Autodesk Inventor part; units mm, degrees
ref_plane "YZ Plane" through (0, 0, 0) normal (1, 0, 0) x (0, 1, 0)
ref_plane "XZ Plane" through (0, 0, 0) normal (0, 1, 0) x (-1, 0, 0)
ref_plane "XY Plane" through (0, 0, 0) normal (0, 0, 1) x (1, 0, 0)
sketch "Sketch1" plane through (0, 0, 0) normal (0, 1, 0) x (-1, 0, 0)
  line L0 (0, 0) -> (152.4, 0)
  line L1 (152.4, 0) -> (152.4, -762)
  line L2 (0, -762) -> (0, 0)
  line L3 (152.4, -762) -> (0, -762) construction
  arc A0 (0, -762) -> (152.4, -762) centre (76.2, -936.5961) ccw
  line L4 (152.4, -590.1365) -> (152.4, -762) construction
  arc A1 (12.7, -770.5221) -> (139.7, -770.5221) centre (76.2, -936.5961) ccw
  line L5 (12.7, -12.7) -> (139.7, -12.7)
  line L6 (139.7, -12.7) -> (139.7, -749.3)
  line L7 (12.7, -749.3) -> (12.7, -12.7)
  line L8 (12.7, -12.7) -> (139.7, -749.3) construction
  line L9 (139.7, -12.7) -> (12.7, -749.3) construction
  line L10 (12.7, -749.3) -> (12.7, -770.5221)
  line L11 (139.7, -749.3) -> (139.7, -770.5221)
  point P0 (76.2, -381)
  dimension "d0" = 762
  dimension "d1" = 381
  dimension "d2" = 355.6
  dimension "d3" = 762
  dimension "d4" = 127
  dimension "d5" = 736.6
extrude "Extrusion1" add sketch "Sketch1" along normal blind 12.7
properties part number "Arm Layer 2 Out"
For this review, take the finished solid that the model builds, in its own axes (mm). Round coordinates to 2 decimals unless told otherwise and drop trailing zeros. Write each loop counter-clockwise with the first axis right and the second up, starting at its lowest first coordinate (ties: lowest second). Pieces come first, ordered by that corner, then holes. Notation, with made-up numbers: (54, 44.25) - (103, 44.25) arc R31 cw to (103, 73.25) - close; hole circle Ø10 at (40, 75). An arc over 180 degrees is marked (long way). Use CSV: the item, a comma, the result in double quotes.
1) Add section C-C on y = 4.75. Write out the cut boundary in (x, z), and give its area (3 significant figures).
Conclusion:
outline,"(-152.4, -762) arc R190.5 ccw (long way) to (0, -762) - (0, 0) - (-152.4, 0) - close; hole (-139.7, -770.52) arc R177.8 ccw (long way) to (-12.7, -770.52) - (-12.7, -12.7) - (-139.7, -12.7) - close"
area,"33,900 mm^2"
2) Add section B-B on x = -76.2. Write out the cut boundary in (y, z), and give its area (3 significant figures).
Conclusion:
outline,"(0, -1127.1) - (12.7, -1127.1) - (12.7, -1114.4) - (0, -1114.4) - close; (0, -12.7) - (12.7, -12.7) - (12.7, 0) - (0, 0) - close"
area,"323 mm^2"
3) Wall thickness on line 1 along X through (y, z) = (1.75, -527); line 2 along Z through (x, y) = (-10.5, 2.75); line 3 along X through (y, z) = (11, -1040): over which ranges is each line inside the solid? List them lowest first. Write a range as from..to.
Conclusion:
line 1,"x = -152.4..-139.7, -12.7..0"
line 2,"z = -1115.41..-1101.81, -771.38..0"
line 3,"x = -236.19..-220.84, 68.44..83.79"
4) Add section A-A on z = -109. Write out the cut boundary in (x, y), and give its area (3 significant figures).
Conclusion:
outline,"(-152.4, 0) - (-139.7, 0) - (-139.7, 12.7) - (-152.4, 12.7) - close; (-12.7, 0) - (0, 0) - (0, 12.7) - (-12.7, 12.7) - close"
area,"323 mm^2"
5) The part is to be moulded in two halves that separate along Z. For faces 1 (the cylindrical face through (-83.479, 6.261, -1126.957)), 2 (the flat face through (-5, 12.7, -603)), 3 (the cylindrical face through (-83.11, 6.26, -1114.26)), say which applies: pulls with the +Z half, pulls with the -Z half, needs draft (parallel to the pull), parting line crosses it, or undercut.
Conclusion:
face 1,"parting line crosses it"
face 2,"needs draft"
face 3,"undercut"
6) Clearance check with flat-ended pins moving along their axes: pin 1 Ø4 at (x, y) = (-71.5, 8) entering from -Z; pin 2 Ø1.5 at (y, z) = (11.5, -912.5) entering from -X; pin 3 Ø6 at (y, z) = (7.5, -619) entering from -X. State where each tip first meets the part, or that it passes through.
Conclusion:
pin 1,"stops at z = -1127.08"
pin 2,"stops at x = -265.26"
pin 3,"stops at x = -152.4"
